```python
from build123d import *

# Parameters (mm, degrees)
SKETCH1_W           = 1
SKETCH1_H           = 10
BOSS_EXTRUDE1_DEPTH = 5
SKETCH2_W           = 4
SKETCH2_H           = 5
BOSS_EXTRUDE2_DEPTH = 1
SKETCH3_R           = 0.428245062
CUT_EXTRUDE1_DEPTH  = 1
SKETCH4_R           = 0.1
CUT_EXTRUDE2_DEPTH  = 1


with BuildPart() as part:
    # Sketch1 → Boss-Extrude1 (new body)
    with BuildSketch(Plane.XY):
        with Locations((0.5, 5)):
            Rectangle(SKETCH1_W, SKETCH1_H)
    extrude(amount=BOSS_EXTRUDE1_DEPTH)

    # Sketch2 → Boss-Extrude2 (add)
    with BuildSketch(Plane(origin=(0, 10, 0), x_dir=(1, 0, 0), z_dir=(0, 1, 0))):
        with Locations((-1, -2.5)):
            Rectangle(SKETCH2_W, SKETCH2_H)
    extrude(amount=BOSS_EXTRUDE2_DEPTH)

    # Sketch3 → Cut-Extrude1 (cut)
    with BuildSketch(Plane(origin=(1, 0, 0), x_dir=(0, 0, -1), z_dir=(1, 0, 0))):
        with Locations((-2.508031341, 5.528987799)):
            Circle(SKETCH3_R)
    extrude(amount=-CUT_EXTRUDE1_DEPTH, mode=Mode.SUBTRACT)

    # Sketch4 → Cut-Extrude2 (cut)
    with BuildSketch(Plane(origin=(0, 10, 0), x_dir=(-1, 0, 0), z_dir=(0, -1, 0))):
        with Locations(Location((1.494110206, -1.366840593, 0), (0, 0, 90))):
            Circle(SKETCH4_R)
        with Locations(Location((1.494110206, -3.646335679, 0), (0, 0, 90))):
            Circle(SKETCH4_R)
    extrude(amount=-CUT_EXTRUDE2_DEPTH, mode=Mode.SUBTRACT)


solid = part.part
```
Here's how the part is built. I have some questions about the finished solid (model axes, mm). A direction names the side the tool comes from. Coordinates: 2 decimals unless noted, no trailing zeros. Order: outer loops, then holes, each group sorted by start corner. A loop starts at its lowest first (then second) coordinate and runs counter-clockwise, first axis right, second up. Notation, with made-up numbers: (-7.75, 7.25) - (40.25, 7.25) arc R27 ccw to (40.25, 40.25) - close; hole circle Ø10 at (31, 79). An arc over 180 degrees is marked (long way). One line per question, with ' | ' between items. Start each with the question number.
1. Which directions (+Z, -Z, +X, -X, +Y, -Y) give clear straight access to the entire face, cutting with the end or side of a thin tool? Please do faces 4 (the flat face through (-2, 10, 2)), 5 (the flat face through (0.3, 6.3, 0)).
2. I'm going to push flat-ended pins straight in: pin 1 Ø2.5 at (y, z) = (7, 2.5) entering from -X; pin 2 Ø2 at (x, z) = (-1.5, 2.5) entering from -Y. Where does each tip first touch, or does it pass through?
3. If we section it at C-C (z = 4.15): Write out the boundary of the cut face in (x, y), and give its area (3 significant figures).
4. If we mould it in two halves opening along Y, with no side actions, what happens to faces 1 (the flat face through (-1, 11, 2)), 2 (the flat face through (0, 5, 2)), 3 (the cylindrical face through (0.51, 5.15, 2.31))? For each: released by +Y, released by -Y, zero draft, split by the parting line, or undercut.
5. If we section it at D-D (x = -0.6): Write out the boundary of the cut face in (y, z).
6. If we section it at A-A (z = 2.65): Write out the boundary of the cut face in (x, y), and give its area (3 significant figures).
7. Please list where these lines run through material, in increasing order: line 1 along Y through (x, z) = (-2.05, 1.05); line 2 along X through (y, z) = (3.5, 4.7); line 3 along Y through (x, z) = (0.8, 2.3). Write a range as [from, to].
8. If we section it at B-B (y = 0.75): Write out the boundary of the cut face in (x, z).
Model answer:
1) face 4: +Z, -Z, -X, -Y | face 5: -Z, +X, -X, +Y, -Y
2) pin 1: stops at x = 0 | pin 2: stops at y = 10
3) outline: (-3, 10) - (0, 10) - (0, 0) - (1, 0) - (1, 11) - (-3, 11) - close | area: 14.0 mm²
4) face 1: released by +Y | face 2: zero draft | face 3: undercut
5) outline: (10, 0) - (11, 0) - (11, 5) - (10, 5) - close
6) outline: (-3, 10) - (0, 10) - (0, 5.93) - (1, 5.93) - (1, 11) - (-3, 11) - close; (0, 0) - (1, 0) - (1, 5.12) - (0, 5.12) - close | area: 13.2 mm²
7) line 1: y = [10, 11] | line 2: x = [0, 1] | line 3: y = [0, 5.15], [5.9, 11]
8) outline: (0, 0) - (1, 0) - (1, 5) - (0, 5) - close
